Here's how the part is built. I have some questions about the finished solid (model axes, mm). Face numbers are marked on the shaded views. Round coordinates to 2 decimals unless told otherwise and drop trailing zeros. Loops run counter-clockwise (first coordinate to the right, second up) from the corner with the lowest first, then second, coordinate; pieces in that order, holes last. Notation, with made-up numbers: (5.5, 39.5) -> (10.5, 39.5) arc R23 ccw to (10.5, 62.5) -> close; hole circle Ø9 at (31.25, 64.5). An arc over 180 degrees is marked (long way). One line per item, written item: value. Start each with the question number.
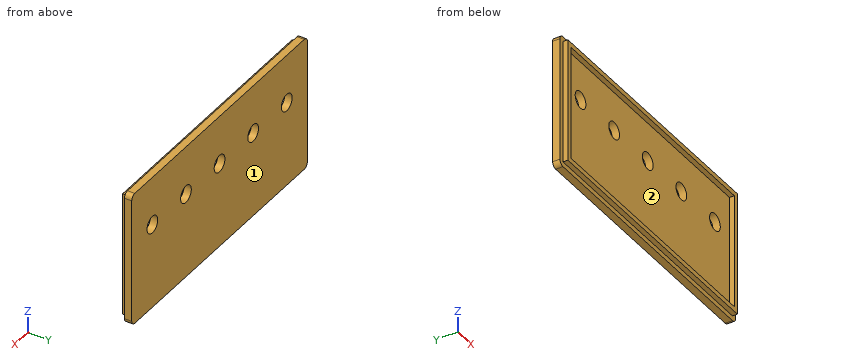
```python
from build123d import *

# Parameters (mm, degrees)
SKETCH_1_W          = 115
SKETCH_1_H          = 55
EXTRUDE_1_DEPTH     = 3
SKETCH_2_R          = 3.5
CUT_EXTRUDE_1_DEPTH = 3
SKETCH_4_W          = 111
SKETCH_4_H          = 51
SKETCH_4_W_2        = 107
SKETCH_4_H_2        = 47
EXTRUDE_2_DEPTH     = 2
FILLET_1_R          = 2


with BuildPart() as part:
    # 草图1 → 凸台-拉伸1 (new body)
    with BuildSketch(Plane(origin=(0, 0, 0), x_dir=(1, 0, 0), z_dir=(0, 1, 0))):
        Rectangle(SKETCH_1_W, SKETCH_1_H)
    extrude(amount=EXTRUDE_1_DEPTH)

    # 草图2 → 切除-拉伸1 (cut)
    with BuildSketch(Plane(origin=(0, 3, 0), x_dir=(1, 0, 0), z_dir=(0, 1, 0))):
        with Locations(Location((-44, -7.5, 0), (0, 0, 270))):
            Circle(SKETCH_2_R)
        with Locations(Location((-22, -7.5, 0), (0, 0, 270))):
            Circle(SKETCH_2_R)
        with Locations(Location((0, -7.5, 0), (0, 0, 270))):
            Circle(SKETCH_2_R)
        with Locations(Location((22, -7.5, 0), (0, 0, 270))):
            Circle(SKETCH_2_R)
        with Locations(Location((44, -7.5, 0), (0, 0, 270))):
            Circle(SKETCH_2_R)
    extrude(amount=-CUT_EXTRUDE_1_DEPTH, mode=Mode.SUBTRACT)

    # 草图4 → 凸台-拉伸2 (add)
    with BuildSketch(Plane.XZ):
        Rectangle(SKETCH_4_W, SKETCH_4_H)
        Rectangle(SKETCH_4_W_2, SKETCH_4_H_2, mode=Mode.SUBTRACT)
    extrude(amount=EXTRUDE_2_DEPTH)

    # 圆角1
    fillet_1_edges = [part.edges().sort_by_distance(p)[0] for p in [
        (57.5, 1.5, 27.5),
        (-57.5, 1.5, 27.5),
        (-57.5, 1.5, -27.5),
        (57.5, 1.5, -27.5),
    ]]
    fillet(fillet_1_edges, radius=FILLET_1_R)


solid = part.part
```
Q1. I want a section at B-B on z = 13.5. Please give me the cut outline in (x, y), plus the area to 3 significant figures.
Q2. If we mould it in two halves opening along Z, with no side actions, what happens to the marked faces 1 and 2? For each: released by +Z, released by -Z, zero draft, split by the parting line, or undercut.
Q3. I want a section at C-C on y = 1.3. Please give me the cut outline in (x, z).
Q4. I want a section at A-A on x = -22. Please give me the cut outline in (y, z).
Q5. Will these pins go through, and if not, where does the flat tip stop? P1, Ø9, axis at x = -44, z = 7.5, coming from the -Y side; P2, Ø1, axis at y = -1, z = 6, coming from the +X side; P3, Ø0.6, axis at x = 9.5, y = -0.5, coming from the +Z side.
Q6. If I drill on line 1 along X through (y, z) = (2.1, 7.5); line 2 along X through (y, z) = (-0.75, 15.5); line 3 along Z through (x, y) = (-32, -1.2), over which ranges is the centre line in solid material (lowest first)?
Q7. I want a section at D-D on x = 30. Please give me the cut outline in (y, z), plus the area to 3 significant figures.
Answers below:
1. outline: (-57.5, 0) -> (-55.5, 0) -> (-55.5, -2) -> (-53.5, -2) -> (-53.5, 0) -> (53.5, 0) -> (53.5, -2) -> (55.5, -2) -> (55.5, 0) -> (57.5, 0) -> (57.5, 3) -> (-57.5, 3) -> close
1. area: 353 mm^2
2. face 1: zero draft
2. face 2: undercut
3. outline: (-57.5, -25.5) arc R2 ccw to (-55.5, -27.5) -> (55.5, -27.5) arc R2 ccw to (57.5, -25.5) -> (57.5, 25.5) arc R2 ccw to (55.5, 27.5) -> (-55.5, 27.5) arc R2 ccw to (-57.5, 25.5) -> close; hole circle Ø7 at (-44, 7.5); hole circle Ø7 at (-22, 7.5); hole circle Ø7 at (0, 7.5); hole circle Ø7 at (22, 7.5); hole circle Ø7 at (44, 7.5)
4. outline: (-2, -25.5) -> (0, -25.5) -> (0, -27.5) -> (3, -27.5) -> (3, 4) -> (0, 4) -> (0, -23.5) -> (-2, -23.5) -> close; (-2, 23.5) -> (0, 23.5) -> (0, 11) -> (3, 11) -> (3, 27.5) -> (0, 27.5) -> (0, 25.5) -> (-2, 25.5) -> close
5. P1: stops at y = 0
5. P2: stops at x = 55.5
5. P3: stops at z = 25.5
6. line 1: x = -57.5 to -47.5, -40.5 to -25.5, -18.5 to -3.5, 3.5 to 18.5, 25.5 to 40.5, 47.5 to 57.5
6. line 2: x = -55.5 to -53.5, 53.5 to 55.5
6. line 3: z = -25.5 to -23.5, 23.5 to 25.5
7. outline: (-2, -25.5) -> (0, -25.5) -> (0, -27.5) -> (3, -27.5) -> (3, 27.5) -> (0, 27.5) -> (0, 25.5) -> (-2, 25.5) -> (-2, 23.5) -> (0, 23.5) -> (0, -23.5) -> (-2, -23.5) -> close
7. area: 173 mm^2
